```python
from build123d import *

# Parameters (mm, degrees)
BOSS_EXTRUDE1_DEPTH = 1.524


with BuildPart() as part:
    # Sketch1 → Boss-Extrude1 (new body)
    with BuildSketch(Plane.XY):
        with BuildLine():
            Line((-277.916022261, 935.884590671), (-285.203156616, 935.884606348))
            Line((-285.203156616, 935.884606348), (-285.203156616, 937.391012124))
            Line((-285.203156616, 937.391012124), (-277.916022261, 937.391027801))
            ThreePointArc((-277.916022261, 937.391027801), (-277.404732191, 937.602812049), (-277.192949044, 938.114102574))
            ThreePointArc((-277.192949044, 938.114102574), (-277.338273323, 939.523325046), (-278.333966376, 940.531106008))
            ThreePointArc((-278.333966376, 940.531106008), (-281.120669571, 941.782213098), (-284.027620805, 942.720625679))
            ThreePointArc((-284.027620805, 942.720625679), (-288.327575015, 944.323536073), (-292.30676806, 946.609351169))
            ThreePointArc((-292.30676806, 946.609351169), (-292.318053521, 944.881271306), (-291.117622598, 943.638149038))
            ThreePointArc((-291.117622598, 943.638149038), (-293.581810552, 943.528926691), (-296.026671847, 943.202116281))
            ThreePointArc((-296.026671847, 943.202116281), (-304.765117762, 946.571977556), (-310.958943201, 953.597141502))
            ThreePointArc((-310.958943201, 953.597141502), (-312.909914326, 961.259205892), (-311.83641056, 969.092539073))
            ThreePointArc((-311.83641056, 969.092539073), (-312.032754546, 970.855390285), (-312.723616891, 972.489068521))
            ThreePointArc((-312.723616891, 972.489068521), (-312.075442701, 972.234238525), (-311.427268511, 972.489068521))
            ThreePointArc((-311.427268511, 972.489068521), (-309.093003832, 975.689484265), (-308.423499884, 979.593740531))
            ThreePointArc((-308.423499884, 979.593740531), (-306.900843126, 981.252159973), (-305.996550373, 983.313977924))
            ThreePointArc((-305.996550373, 983.313977924), (-307.073192817, 982.682922072), (-308.296117566, 982.434234514))
            ThreePointArc((-308.296117566, 982.434234514), (-307.955705891, 983.149057367), (-307.497960974, 983.795061554))
            ThreePointArc((-307.497960974, 983.795061554), (-307.339448033, 985.49236907), (-307.429564156, 987.194678748))
            ThreePointArc((-307.429564156, 987.194678748), (-306.664530959, 989.110784639), (-306.404290892, 991.157492406))
            ThreePointArc((-306.404290892, 991.157492406), (-306.936605496, 990.101048934), (-307.973845227, 989.532220851))
            ThreePointArc((-307.973845227, 989.532220851), (-308.148188947, 990.005120957), (-308.342762435, 990.47006332))
            ThreePointArc((-308.342762435, 990.47006332), (-312.267081574, 995.727304596), (-313.766747643, 1002.113999219))
            ThreePointArc((-313.766747643, 1002.113999219), (-315.73298932, 997.693682682), (-315.365124744, 992.869785889))
            ThreePointArc((-315.365124744, 992.869785889), (-312.991611752, 988.301516567), (-311.716030786, 983.313977924))
            ThreePointArc((-311.716030786, 983.313977924), (-311.804694988, 981.790848195), (-312.68001538, 980.541208357))
            ThreePointArc((-312.68001538, 980.541208357), (-314.117806981, 978.199671225), (-314.619350909, 975.498098624))
            ThreePointArc((-314.619350909, 975.498098624), (-315.225884586, 975.805286829), (-315.64332213, 976.341937173))
            ThreePointArc((-315.64332213, 976.341937173), (-315.299209722, 974.750720167), (-315.381025476, 973.124777027))
            ThreePointArc((-315.381025476, 973.124777027), (-315.973449697, 972.588843997), (-316.436986467, 971.938210203))
            ThreePointArc((-316.436986467, 971.938210203), (-317.393086767, 971.150910263), (-318.584467297, 970.812411499))
            ThreePointArc((-318.584467297, 970.812411499), (-317.350697798, 969.220806246), (-316.518624321, 967.386944694))
            ThreePointArc((-316.518624321, 967.386944694), (-316.709257262, 965.229666664), (-317.275247771, 963.139249442))
            ThreePointArc((-317.275247771, 963.139249442), (-317.856536979, 960.284878164), (-317.558763157, 957.387178511))
            ThreePointArc((-317.558763157, 957.387178511), (-317.339657536, 956.598381541), (-317.094041757, 955.817432873))
            ThreePointArc((-317.094041757, 955.817432873), (-318.118043569, 955.930405975), (-319.022729617, 956.423240417))
            ThreePointArc((-319.022729617, 956.423240417), (-317.621338919, 954.158054516), (-315.64332213, 952.374122723))
            ThreePointArc((-315.64332213, 952.374122723), (-313.785435132, 949.339402014), (-311.503309748, 946.609351169))
            ThreePointArc((-311.503309748, 946.609351169), (-312.953347628, 945.841313107), (-314.591537057, 945.747357192))
            ThreePointArc((-314.591537057, 945.747357192), (-311.553116659, 944.299676635), (-308.227229789, 943.78367854))
            ThreePointArc((-308.227229789, 943.78367854), (-304.724383034, 941.692906178), (-300.920541819, 940.219116344))
            ThreePointArc((-300.920541819, 940.219116344), (-300.33247451, 939.844426317), (-300.035650029, 939.213465936))
            ThreePointArc((-300.035650029, 939.213465936), (-302.045043086, 937.407911663), (-304.647627414, 936.683866421))
            ThreePointArc((-304.647627414, 936.683866421), (-302.200371512, 935.891549854), (-299.94034594, 934.663090898))
            ThreePointArc((-299.94034594, 934.663090898), (-300.038049245, 933.69975054), (-300.79307234, 933.093523928))
            ThreePointArc((-300.79307234, 933.093523928), (-308.644427917, 929.185810881), (-314.591537057, 922.740200085))
            ThreePointArc((-314.591537057, 922.740200085), (-316.523960255, 920.558055545), (-319.022728662, 919.057332166))
            ThreePointArc((-319.022728662, 919.057332166), (-317.841309798, 918.862286718), (-316.819146135, 918.238608351))
            ThreePointArc((-316.819146135, 918.238608351), (-317.206321698, 917.112560154), (-317.537734191, 915.968857736))
            ThreePointArc((-317.537734191, 915.968857736), (-318.596134624, 912.830665778), (-319.922253722, 909.795889281))
            ThreePointArc((-319.922253722, 909.795889281), (-318.307455112, 909.712246343), (-316.897931891, 908.919898577))
            ThreePointArc((-316.897931891, 908.919898577), (-316.598343369, 907.286884178), (-316.521377997, 905.628401245))
            ThreePointArc((-316.521377997, 905.628401245), (-317.288501726, 903.611397757), (-318.584467297, 901.885925322))
            ThreePointArc((-318.584467297, 901.885925322), (-317.459455632, 901.812397156), (-316.436986467, 901.337408268))
            ThreePointArc((-316.436986467, 901.337408268), (-315.973449697, 900.686774475), (-315.381025476, 900.150841445))
            ThreePointArc((-315.381025476, 900.150841445), (-314.855793688, 899.575963976), (-314.600768516, 898.84022306))
            ThreePointArc((-314.600768516, 898.84022306), (-315.008341261, 896.492487869), (-315.677043026, 894.205390577))
            ThreePointArc((-315.677043026, 894.205390577), (-315.022224116, 894.879239219), (-314.227435144, 895.380408141))
            ThreePointArc((-314.227435144, 895.380408141), (-313.589841267, 893.977791631), (-312.679998267, 892.734391155))
            ThreePointArc((-312.679998267, 892.734391155), (-311.804692825, 891.484757082), (-311.716030786, 889.961640548))
            ThreePointArc((-311.716030786, 889.961640548), (-311.763791905, 889.630867843), (-311.816449784, 889.300839277))
            ThreePointArc((-311.816449784, 889.300839277), (-312.878083338, 887.113343117), (-314.444692648, 885.253789266))
            ThreePointArc((-314.444692648, 885.253789266), (-313.65384255, 885.493842794), (-312.832184374, 885.404694518))
            ThreePointArc((-312.832184374, 885.404694518), (-313.94276822, 882.826275412), (-315.365124744, 880.405832583))
            ThreePointArc((-315.365124744, 880.405832583), (-317.025672215, 877.438104616), (-319.293323049, 874.903822293))
            ThreePointArc((-319.293323049, 874.903822293), (-315.812908434, 875.83934739), (-312.728096674, 877.702792989))
            ThreePointArc((-312.728096674, 877.702792989), (-308.443902691, 882.584048211), (-307.427457693, 888.998704102))
            ThreePointArc((-307.427457693, 888.998704102), (-308.20314369, 889.43695462), (-309.093003832, 889.480557515))
            ThreePointArc((-309.093003832, 889.480557515), (-308.513125406, 892.598000293), (-308.54961586, 895.768706352))
            ThreePointArc((-308.54961586, 895.768706352), (-309.481516734, 898.387713723), (-311.193435925, 900.577912695))
            ThreePointArc((-311.193435925, 900.577912695), (-310.219823691, 900.257804208), (-309.354771115, 899.708191378))
            ThreePointArc((-309.354771115, 899.708191378), (-310.941483354, 902.250655609), (-312.100693339, 905.014351016))
            ThreePointArc((-312.100693339, 905.014351016), (-313.022128407, 916.44457007), (-307.699732777, 926.601885411))
            ThreePointArc((-307.699732777, 926.601885411), (-302.18443266, 929.41780767), (-296.026671847, 930.073502191))
            ThreePointArc((-296.026671847, 930.073502191), (-295.073187001, 929.919785137), (-294.114945931, 929.799218415))
            ThreePointArc((-294.114945931, 929.799218415), (-293.879713809, 928.583729022), (-294.369589284, 927.446728303))
            ThreePointArc((-294.369589284, 927.446728303), (-291.413219904, 928.960043614), (-288.197659122, 929.790953956))
            ThreePointArc((-288.197659122, 929.790953956), (-283.128142335, 930.80796962), (-278.333966376, 932.744512464))
            ThreePointArc((-278.333966376, 932.744512464), (-277.338273323, 933.752293426), (-277.192949044, 935.161515898))
            ThreePointArc((-277.192949044, 935.161515898), (-277.404732191, 935.672806423), (-277.916022261, 935.884590671))
        make_face()
    extrude(amount=BOSS_EXTRUDE1_DEPTH)


solid = part.part
```
Geometry check sheet. Reference: the model listing, model coordinates, mm. A direction names the side the tool comes from. Round coordinates to 2 decimals unless told otherwise and drop trailing zeros. Loops run counter-clockwise (first coordinate to the right, second up) from the corner with the lowest first, then second, coordinate; pieces in that order, holes last. Notation, with made-up numbers: (52, -7) -> (83, -7) arc R25 cw to (83, 32) -> close; hole circle Ø5 at (39.5, 75). An arc over 180 degrees is marked (long way). Use a Markdown table: item, result.
(1) Scan lines: probe 1 along Y at (x, z) = (-303, 0.5); probe 2 along Y at (x, z) = (-304, 0.8); probe 3 along Y at (x, z) = (-314, 1.1). Record each from-to range of solid material in increasing order.
Calculated:
| item | result |
|---|---|
| probe 1 | 929.15 to 932.34, 936.21 to 936.99, 940.93 to 945.48 |
| probe 2 | 928.76 to 931.92, 936.52 to 936.75, 941.35 to 946.07 |
| probe 3 | 876.79 to 882.71, 885.43 to 885.69, 894.79 to 923.63, 945.38 to 945.7, 949.64 to 978.49, 990.56 to 1001.8 |
(2) Set-up check for faces 1 (the cylindrical face through (-310.92, 902.21, 0.75)), 2 (the cylindrical face through (-317.365, 969.245, 0.751)), 3 (the cylindrical face through (-315.86, 875.82, 0.75)): record each of +Z, -Z, +X, -X, +Y, -Y from which the full face is reachable in a straight line by a thin tool's end or side.
Calculated:
| item | result |
|---|---|
| face 1 | +Z, -Z, +X |
| face 2 | +Z, -Z, -X |
| face 3 | +Z, -Z, +X, -Y |
(3) Sectioned sample at C-C (x = -298). Enter the section's corners in (y, z), then the cut area to 3 significant figures.
Calculated:
| item | result |
|---|---|
| outline | (930.11, 0) -> (943.56, 0) -> (943.56, 1.52) -> (930.11, 1.52) -> close |
| area | 20.5 mm² |
(4) Sectioned sample at A-A (x = -279.5). Enter the section's corners in (y, z).
Calculated:
| item | result |
|---|---|
| outline | (932.18, 0) -> (935.88, 0) -> (935.88, 1.52) -> (932.18, 1.52) -> close; (937.39, 0) -> (941.1, 0) -> (941.1, 1.52) -> (937.39, 1.52) -> close |
(5) Go/stop test with a flat-tipped pin: P1, Ø0.8, axis at x = -281, z = 1, coming from the +Y side. Record where the tip stops, or that it passes through.
Calculated:
| item | result |
|---|---|
| P1 | y = 941.89 |
(6) Sectioned sample at B-B (y = 891.5). Enter the section's corners in (x, z).
Calculated:
| item | result |
|---|---|
| outline | (-311.81, 0) -> (-308.65, 0) -> (-308.65, 1.52) -> (-311.81, 1.52) -> close |
(7) Mould release check, pull along Y, two halves, no side actions. Record for faces 4 (the cylindrical face through (-309.46, 898.35, 0.75)), 5 (the flat face through (-300, 939, 1.524)), 6 (the cylindrical face through (-304.66, 946.5, 0.75)), 7 (the cylindrical face through (-283.198, 930.787, 0.751)): released by +Y, released by -Y, zero draft, split by the parting line, or undercut.
Calculated:
| item | result |
|---|---|
| face 4 | undercut |
| face 5 | zero draft |
| face 6 | undercut |
| face 7 | released by -Y |
